from build123d import *

# Parameters (mm, degrees)
F0_W          = 70
F0_H          = 50
F1_DEPTH      = 9
F2_W          = 35
F2_H          = 35
F3_DEPTH      = 8
F5_DEPTH      = 25
F5_DEPTH_BACK = 25
F6_W          = 0.9375
F6_H          = 1.5
F7_DEPTH      = 25
F7_DEPTH_BACK = 25
F8_SIZE       = 2


with BuildPart() as f1:
    # F0 (on Top) → F1 (new body)
    with BuildSketch(Plane.XY):
        Rectangle(F0_W, F0_H)
    extrude(amount=F1_DEPTH)

    # F2 (on face) → F3 (join)
    with BuildSketch(Plane(origin=(0, 0, 0), x_dir=(1, 0, 0), z_dir=(0, 0, -1))):
        Rectangle(F2_W, F2_H)
    extrude(amount=F3_DEPTH)

    # F4 (on Front) → F5 (cut, two sides)
    with BuildSketch(Plane.XZ) as f5_sk:
        Polygon((12.5, 0), (16.5625, -6.5), (16.5625, -8), (17.5, -8), (17.5, 0), align=None)
        Polygon((-16.5625, -6.5), (-12.5, 0), (-17.5, 0), (-17.5, -8), (-16.5625, -8), align=None)
    extrude(amount=-F5_DEPTH, mode=Mode.SUBTRACT)
    extrude(f5_sk.sketch, amount=F5_DEPTH_BACK, mode=Mode.SUBTRACT)

    # F6 (on Right) → F7 (cut, two sides)
    with BuildSketch(Plane.YZ) as f7_sk:
        Polygon((17.5, 0), (12.5, 0), (16.5625, -6.5), (17.5, -6.5), align=None)
        with Locations((17.03125, -7.25)):
            Rectangle(F6_W, F6_H)
        Polygon((-17.5, 0), (-17.5, -8), (-16.5625, -8), (-16.5625, -6.5), (-12.5, 0), align=None)
    extrude(amount=-F7_DEPTH, mode=Mode.SUBTRACT)
    extrude(f7_sk.sketch, amount=F7_DEPTH_BACK, mode=Mode.SUBTRACT)

    # F8
    f8_edges = [f1.edges().sort_by_distance(p)[0] for p in [
        (35, 0, 9),
        (0, 25, 9),
        (-35, 0, 9),
        (0, -25, 9),
        (0, -25, 0),
        (35, 0, 0),
        (0, 25, 0),
        (-35, 0, 0),
    ]]
    chamfer(f8_edges, length=F8_SIZE)


solid = f1.part
For this review, take the finished solid that the model builds, in its own axes (mm). A direction names the side the tool comes from. Give positions to 0.01 mm unless a question says otherwise; leave off trailing zeros. Order: outer loops, then holes, each group sorted by start corner. A loop starts at its lowest first (then second) coordinate and runs counter-clockwise, first axis right, second up. Notation, with made-up numbers: M 84,-0.5 L 124,-0.5 A27 cw 124,18.5 Z; hole C 38.5,37.25 d9. An arc over 180 degrees is marked long. Answer in a Markdown table with one row per item. Add a question column.
(1) Consider section C-C on x = -14. State the section outline as (y, z) points, and give its area (3 significant figures).
(2) Wall thickness on probe 1 along Z at (x, y) = (3, -19.5); probe 2 along Z at (x, y) = (-14.5, -15); probe 3 along Y at (x, z) = (16, 1): over which ranges is each line inside the solid? List them lowest first. Write a range as [from, to].
(3) Mouldability with a two-part tool opening along Z and no side actions: class faces 5 (the face through (14, 0, 0)), 6 (the face through (0, -16.562, -7)), 7 (the face through (34, 0, 1)) as +Z half, -Z half, draft (parallel to the pull), parting line (faces both ways), or undercut.
(4) Consider section B-B on x = -4.5. State the section outline as (y, z) points.
(5) Consider section D-D on y = 7. State the section outline as (x, z) points.
(6) For faces 1 (the face through (16.562, 0, -7)), 2 (the face through (-14.56, -0.232, -3.295)), 3 (the face through (0.232, -14.56, -3.295)), 4 (the face through (0, 16.562, -7)), list the 3-axis set-ups (+Z, -Z, +X, -X, +Y, -Y) from which the entire face can be reached by the end or side of a thin tool; tool diameter is ignored.
(7) For pin 1 (1.5 mm diameter, centred on x = 27.5, z = 0.5, fed in from +Y); pin 2 (0.8 mm diameter, centred on x = 1, z = -7.5, fed in from +Y); pin 3 (1.5 mm diameter, centred on x = 21.5, y = -13.5, fed in from -Z), all flat-tipped, find the tip position at first contact; note any pin that passes through.
(8) Consider section A-A on y = -13.5. State the section outline as (x, z) points, and give its area (3 significant figures).
Evaluation:
| question | item | result |
|---|---|---|
| 1 | outline | M -25,2 L -23,0 L 23,0 L 25,2 L 25,7 L 23,9 L -23,9 L -25,7 Z; M -16.56,-8 L 16.56,-8 L 16.56,-6.5 L 14,-2.4 L -14,-2.4 L -16.56,-6.5 Z |
| 1 | area | 617 mm^2 |
| 2 | probe 1 | z = [0, 9] |
| 2 | probe 2 | z = [-8, -4], [0, 9] |
| 2 | probe 3 | y = [-24, 24] |
| 3 | face 5 | undercut |
| 3 | face 6 | draft |
| 3 | face 7 | -Z half |
| 4 | outline | M -25,2 L -23,0 L -12.5,0 L -16.56,-6.5 L -16.56,-8 L 16.56,-8 L 16.56,-6.5 L 12.5,0 L 23,0 L 25,2 L 25,7 L 23,9 L -23,9 L -25,7 Z |
| 5 | outline | M -35,2 L -33,0 L -12.5,0 L -16.56,-6.5 L -16.56,-8 L 16.56,-8 L 16.56,-6.5 L 12.5,0 L 33,0 L 35,2 L 35,7 L 33,9 L -33,9 L -35,7 Z |
| 6 | face 1 | -Z, +X, +Y, -Y |
| 6 | face 2 | -X, +Y, -Y |
| 6 | face 3 | +X, -X, -Y |
| 6 | face 4 | -Z, +X, -X, +Y |
| 7 | pin 1 | stops at y = 24.25 |
| 7 | pin 2 | stops at y = 16.56 |
| 7 | pin 3 | stops at z = 0 |
| 8 | outline | M -35,2 L -33,0 L 33,0 L 35,2 L 35,7 L 33,9 L -33,9 L -35,7 Z; M -16.56,-8 L 16.56,-8 L 16.56,-6.5 L 13.5,-1.6 L -13.5,-1.6 L -16.56,-6.5 Z |
| 8 | area | 819 mm^2 |
